Design review of the part built by this model. Coordinates are the model's own, in mm. Face numbers are marked on the shaded views. Round coordinates to 2 decimals unless told otherwise and drop trailing zeros. Write each loop counter-clockwise with the first axis right and the second up, starting at its lowest first coordinate (ties: lowest second). Pieces come first, ordered by that corner, then holes. Notation, with made-up numbers: (-10.75, -7) -> (33.25, -7) arc R18 ccw to (33.25, 18) -> close; hole circle Ø6 at (79.25, 74). An arc over 180 degrees is marked (long way). Write item = value, one per line. Start each with the question number.
Item 1: Add section C-C, the plane z = 124. State the section outline as (x, y) points.
Item 2: For pin 1 Ø1.5 at (x, z) = (16, 61.5) entering from +Y; pin 2 Ø3.5 at (x, z) = (-9.05, 111.48) entering from +Y; pin 3 Ø3 at (x, z) = (46.5, 136.5) entering from +Y; pin 4 Ø8 at (y, z) = (7.5, 117) entering from -X, all flat-tipped, find the tip position at first contact; note any pin that passes through.
Item 3: Add section B-B, the plane y = 19. State the section outline as (x, z) points (3 decimals).
Item 4: To check wall thickness, follow L1, parallel to Z at x = -45, y = 22 (3 decimals); L2, parallel to X at y = 1, z = 25 (3 decimals); L3, parallel to Y at x = 0, z = 69. State the ranges of each line that lie inside material, in increasing order.
Item 5: Add section A-A, the plane y = 7.5. State how many separate pieces and enclosed holes the cut face has, then the cut area to 3 significant figures.
Item 6: Mouldability with a two-part tool opening along Y and no side actions: class the marked faces 1 and 2 as released by +Y, released by -Y, zero draft, split by the parting line, or undercut.
Item 7: Add section D-D, the plane x = -27. State the section outline as (y, z) points.
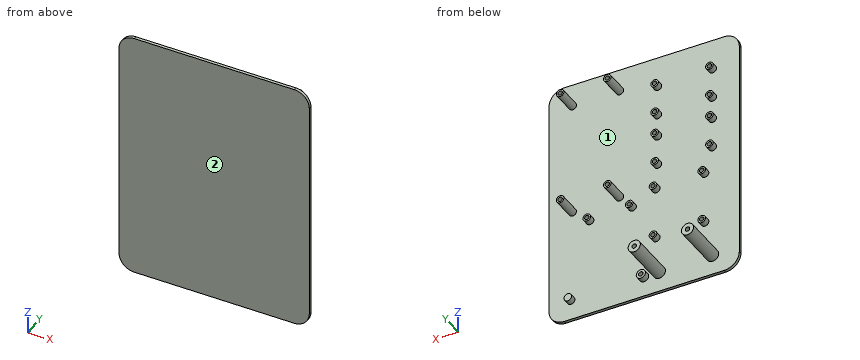
from build123d import *

# Parameters (mm, degrees)
SKETCH_1_R         = 2.5
EXTRUDE_1_DEPTH    = 4
SKETCH_1_R_2       = 3
EXTRUDE_1_2_DEPTH  = 4
EXTRUDE_1_3_DEPTH  = 4
EXTRUDE_1_4_DEPTH  = 4
EXTRUDE_1_5_DEPTH  = 4
EXTRUDE_1_6_DEPTH  = 4
EXTRUDE_1_7_DEPTH  = 4
EXTRUDE_1_8_DEPTH  = 4
EXTRUDE_1_9_DEPTH  = 4
EXTRUDE_1_10_DEPTH = 4
EXTRUDE_1_11_DEPTH = 4
EXTRUDE_1_12_DEPTH = 4
EXTRUDE_1_13_DEPTH = 4
EXTRUDE_1_14_DEPTH = 4
EXTRUDE_1_15_DEPTH = 4
EXTRUDE_1_16_DEPTH = 4
SKETCH_1_3_R       = 2.5
EXTRUDE_2_DEPTH    = 15
EXTRUDE_2_2_DEPTH  = 15
EXTRUDE_2_3_DEPTH  = 15
EXTRUDE_2_4_DEPTH  = 15
SKETCH_1_4_R       = 4
EXTRUDE_3_DEPTH    = 30
EXTRUDE_3_2_DEPTH  = 30
SKETCH_2_W         = 125
SKETCH_2_H         = 165
EXTRUDE_4_DEPTH    = 2
FILLET_1_R         = 10
SKETCH_9_W         = 1.475
SKETCH_9_H         = 30
MM_3_AT_2_COUNT    = 2
MM_3_AT_2_PITCH    = 56.007567425
MM_3_AT_3_COUNT    = 2
MM_3_AT_3_PITCH    = 72.159569674
MM_3_AT_4_COUNT    = 2
MM_3_AT_4_PITCH    = 52.22731905
MM_3_AT_5_COUNT    = 2
MM_3_AT_5_PITCH    = 37.325726715
MM_3_AT_6_COUNT    = 2
MM_3_AT_6_PITCH    = 17.717201651
MM_3_AT_7_COUNT    = 2
MM_3_AT_7_PITCH    = 34.5
MM_3_AT_8_COUNT    = 2
MM_3_AT_8_PITCH    = 59.709714453
MM_3_AT_9_COUNT    = 2
MM_3_AT_9_PITCH    = 66.635200908
MM_3_AT_10_COUNT   = 2
MM_3_AT_10_PITCH   = 71.695536821
MM_3_AT_11_COUNT   = 2
MM_3_AT_11_PITCH   = 75.871602066
MM_3_AT_12_COUNT   = 2
MM_3_AT_12_PITCH   = 86.987675624
MM_3_AT_13_COUNT   = 2
MM_3_AT_13_PITCH   = 116.476846242
MM_3_AT_14_COUNT   = 2
MM_3_AT_14_PITCH   = 95.586858976
MM_3_AT_15_COUNT   = 2
MM_3_AT_15_PITCH   = 78.355146818
MM_3_AT_16_COUNT   = 2
MM_3_AT_16_PITCH   = 60.49973878
MM_3_AT_17_COUNT   = 2
MM_3_AT_17_PITCH   = 48.22587907
MM_3_AT_18_COUNT   = 2
MM_3_AT_18_PITCH   = 35.304741489
MM_3_AT_19_COUNT   = 2
MM_3_AT_19_PITCH   = 32
MM_3_AT_20_COUNT   = 2
MM_3_AT_20_PITCH   = 48.187238975


with BuildPart() as part:
    # Sketch 1 → Extrude 1 (new body)
    with BuildSketch(Plane(origin=(0, 0, 0), x_dir=(1, 0, 0), z_dir=(0, 1, 0))):
        with Locations((-8, -25)):
            Circle(SKETCH_1_R)
    extrude(amount=EXTRUDE_1_DEPTH)



with BuildPart() as body_2:
    # Sketch 1 → Extrude 1 2 (new body)
    with BuildSketch(Plane(origin=(0, 0, 0), x_dir=(1, 0, 0), z_dir=(0, 1, 0))):
        Circle(SKETCH_1_R_2)
    extrude(amount=EXTRUDE_1_2_DEPTH)


with BuildPart() as body_3:
    # Sketch 1 → Extrude 1 3 (new body)
    with BuildSketch(Plane(origin=(0, 0, 0), x_dir=(1, 0, 0), z_dir=(0, 1, 0))):
        with Locations((-9.048256427, -96.482766011)):
            Circle(SKETCH_1_R)
    extrude(amount=EXTRUDE_1_3_DEPTH)


with BuildPart() as body_4:
    # Sketch 1 → Extrude 1 4 (new body)
    with BuildSketch(Plane(origin=(0, 0, 0), x_dir=(1, 0, 0), z_dir=(0, 1, 0))):
        with Locations((-45.048256427, -96.482766011)):
            Circle(SKETCH_1_R)
    extrude(amount=EXTRUDE_1_4_DEPTH)


with BuildPart() as body_5:
    # Sketch 1 → Extrude 1 5 (new body)
    with BuildSketch(Plane(origin=(0, 0, 0), x_dir=(1, 0, 0), z_dir=(0, 1, 0))):
        with Locations((-45.048256427, -76.482766011)):
            Circle(SKETCH_1_R)
    extrude(amount=EXTRUDE_1_5_DEPTH)


with BuildPart() as body_6:
    # Sketch 1 → Extrude 1 6 (new body)
    with BuildSketch(Plane(origin=(0, 0, 0), x_dir=(1, 0, 0), z_dir=(0, 1, 0))):
        with Locations((-9.048256427, -76.482766011)):
            Circle(SKETCH_1_R)
    extrude(amount=EXTRUDE_1_6_DEPTH)


with BuildPart() as body_7:
    # Sketch 1 → Extrude 1 7 (new body)
    with BuildSketch(Plane(origin=(0, 0, 0), x_dir=(1, 0, 0), z_dir=(0, 1, 0))):
        with Locations((-45.048256427, -131.482766011)):
            Circle(SKETCH_1_R)
    extrude(amount=EXTRUDE_1_7_DEPTH)


with BuildPart() as body_8:
    # Sketch 1 → Extrude 1 8 (new body)
    with BuildSketch(Plane(origin=(0, 0, 0), x_dir=(1, 0, 0), z_dir=(0, 1, 0))):
        with Locations((-45.048256427, -111.482766011)):
            Circle(SKETCH_1_R)
    extrude(amount=EXTRUDE_1_8_DEPTH)


with BuildPart() as body_9:
    # Sketch 1 → Extrude 1 9 (new body)
    with BuildSketch(Plane(origin=(0, 0, 0), x_dir=(1, 0, 0), z_dir=(0, 1, 0))):
        with Locations((-9.048256427, -111.482766011)):
            Circle(SKETCH_1_R)
    extrude(amount=EXTRUDE_1_9_DEPTH)


with BuildPart() as body_10:
    # Sketch 1 → Extrude 1 10 (new body)
    with BuildSketch(Plane(origin=(0, 0, 0), x_dir=(1, 0, 0), z_dir=(0, 1, 0))):
        with Locations((-40, -59.5)):
            Circle(SKETCH_1_R)
    extrude(amount=EXTRUDE_1_10_DEPTH)


with BuildPart() as body_11:
    # Sketch 1 → Extrude 1 11 (new body)
    with BuildSketch(Plane(origin=(0, 0, 0), x_dir=(1, 0, 0), z_dir=(0, 1, 0))):
        with Locations((-8, -59.5)):
            Circle(SKETCH_1_R)
    extrude(amount=EXTRUDE_1_11_DEPTH)


with BuildPart() as body_12:
    # Sketch 1 → Extrude 1 12 (new body)
    with BuildSketch(Plane(origin=(0, 0, 0), x_dir=(1, 0, 0), z_dir=(0, 1, 0))):
        with Locations((48, 0)):
            Circle(SKETCH_1_R)
    extrude(amount=EXTRUDE_1_12_DEPTH)


with BuildPart() as body_13:
    # Sketch 1 → Extrude 1 13 (new body)
    with BuildSketch(Plane(origin=(0, 0, 0), x_dir=(1, 0, 0), z_dir=(0, 1, 0))):
        with Locations((-9.048256427, -131.482766011)):
            Circle(SKETCH_1_R)
    extrude(amount=EXTRUDE_1_13_DEPTH)


with BuildPart() as body_14:
    # Sketch 1 → Extrude 1 14 (new body)
    with BuildSketch(Plane(origin=(0, 0, 0), x_dir=(1, 0, 0), z_dir=(0, 1, 0))):
        with Locations((7.6, -52)):
            Circle(SKETCH_1_R)
    extrude(amount=EXTRUDE_1_14_DEPTH)


with BuildPart() as body_15:
    # Sketch 1 → Extrude 1 15 (new body)
    with BuildSketch(Plane(origin=(0, 0, 0), x_dir=(1, 0, 0), z_dir=(0, 1, 0))):
        with Locations((35.5, -52)):
            Circle(SKETCH_1_R)
    extrude(amount=EXTRUDE_1_15_DEPTH)


with BuildPart() as body_16:
    # Sketch 1 → Extrude 1 16 (new body)
    with BuildSketch(Plane(origin=(0, 0, 0), x_dir=(1, 0, 0), z_dir=(0, 1, 0))):
        with Locations((-40, -25)):
            Circle(SKETCH_1_R)
    extrude(amount=EXTRUDE_1_16_DEPTH)


with BuildPart() as body_17:
    # Sketch 1_3 → Extrude 2 (new body)
    with BuildSketch(Plane(origin=(0, 0, 0), x_dir=(1, 0, 0), z_dir=(0, 1, 0))):
        with Locations((15.951743573, -137)):
            Circle(SKETCH_1_3_R)
    extrude(amount=EXTRUDE_2_DEPTH)


with BuildPart() as body_18:
    # Sketch 1_3 → Extrude 2 2 (new body)
    with BuildSketch(Plane(origin=(0, 0, 0), x_dir=(1, 0, 0), z_dir=(0, 1, 0))):
        with Locations((46.951743573, -137)):
            Circle(SKETCH_1_3_R)
    extrude(amount=EXTRUDE_2_2_DEPTH)


with BuildPart() as body_19:
    # Sketch 1_3 → Extrude 2 3 (new body)
    with BuildSketch(Plane(origin=(0, 0, 0), x_dir=(1, 0, 0), z_dir=(0, 1, 0))):
        with Locations((46.951743573, -62)):
            Circle(SKETCH_1_3_R)
    extrude(amount=EXTRUDE_2_3_DEPTH)


with BuildPart() as body_20:
    # Sketch 1_3 → Extrude 2 4 (new body)
    with BuildSketch(Plane(origin=(0, 0, 0), x_dir=(1, 0, 0), z_dir=(0, 1, 0))):
        with Locations((15.951743573, -62)):
            Circle(SKETCH_1_3_R)
    extrude(amount=EXTRUDE_2_4_DEPTH)


with BuildPart() as body_21:
    # Sketch 1_4 → Extrude 3 (new body)
    with BuildSketch(Plane(origin=(0, 0, 0), x_dir=(1, 0, 0), z_dir=(0, 1, 0))):
        with Locations((-45, 0)):
            Circle(SKETCH_1_4_R)
    extrude(amount=EXTRUDE_3_DEPTH)


with BuildPart() as body_22:
    # Sketch 1_4 → Extrude 3 2 (new body)
    with BuildSketch(Plane(origin=(0, 0, 0), x_dir=(1, 0, 0), z_dir=(0, 1, 0))):
        with Locations((-10, 0)):
            Circle(SKETCH_1_4_R)
    extrude(amount=EXTRUDE_3_2_DEPTH)


with BuildPart() as part_1:
    add(part.part)

    add(body_2.part)  # Extrude 4 merges body 2

    add(body_3.part)  # Extrude 4 merges body 3

    add(body_4.part)  # Extrude 4 merges body 4

    add(body_5.part)  # Extrude 4 merges body 5

    add(body_6.part)  # Extrude 4 merges body 6

    add(body_7.part)  # Extrude 4 merges body 7

    add(body_8.part)  # Extrude 4 merges body 8

    add(body_9.part)  # Extrude 4 merges body 9

    add(body_10.part)  # Extrude 4 merges body 10

    add(body_11.part)  # Extrude 4 merges body 11

    add(body_12.part)  # Extrude 4 merges body 12

    add(body_13.part)  # Extrude 4 merges body 13

    add(body_14.part)  # Extrude 4 merges body 14

    add(body_15.part)  # Extrude 4 merges body 15

    add(body_16.part)  # Extrude 4 merges body 16

    add(body_17.part)  # Extrude 4 merges body 17

    add(body_18.part)  # Extrude 4 merges body 18

    add(body_19.part)  # Extrude 4 merges body 19

    add(body_20.part)  # Extrude 4 merges body 20

    add(body_21.part)  # Extrude 4 merges body 21

    add(body_22.part)  # Extrude 4 merges body 22
    # Sketch 2 → Extrude 4 (add)
    with BuildSketch(Plane(origin=(0, 0, 0), x_dir=(1, 0, 0), z_dir=(0, 1, 0))):
        with Locations((0, -69.425835086)):
            Rectangle(SKETCH_2_W, SKETCH_2_H)
    extrude(amount=-EXTRUDE_4_DEPTH)

    # Fillet 1
    fillet_1_edges = [part_1.edges().sort_by_distance(p)[0] for p in [
        (62.5, -1, -13.074164914),
        (62.5, -1, 151.925835086),
        (-62.5, -1, 151.925835086),
        (-62.5, -1, -13.074164914),
    ]]
    fillet(fillet_1_edges, radius=FILLET_1_R)

    # Sketch 9 → mm _3 (revolve, cut)
    with BuildSketch(Plane(origin=(-40, 0, 59.5), x_dir=(0, 0, -1), z_dir=(1, 0, 0))):
        with Locations((0.7375, 15)):
            Rectangle(SKETCH_9_W, SKETCH_9_H)
    mm_3 = revolve(axis=Axis((-40, -6.35, 59.5), (0, 1, 0)), mode=Mode.SUBTRACT)

    # mm _3 at 2: mm _3 ×2
    with Locations(*[Vector(0.99900328, 0, 0.044636825) * (i * MM_3_AT_2_PITCH) for i in range(1, MM_3_AT_2_COUNT)]):
        add(mm_3, mode=Mode.SUBTRACT)

    # mm _3 at 3: mm _3 ×2
    with Locations(*[Vector(-0.069959625, 0, 0.997549824) * (i * MM_3_AT_3_PITCH) for i in range(1, MM_3_AT_3_COUNT)]):
        add(mm_3, mode=Mode.SUBTRACT)

    # mm _3 at 4: mm _3 ×2
    with Locations(*[Vector(-0.096659306, 0, 0.995317526) * (i * MM_3_AT_4_PITCH) for i in range(1, MM_3_AT_4_COUNT)]):
        add(mm_3, mode=Mode.SUBTRACT)

    # mm _3 at 5: mm _3 ×2
    with Locations(*[Vector(-0.135248711, 0, 0.99081168) * (i * MM_3_AT_5_PITCH) for i in range(1, MM_3_AT_5_COUNT)]):
        add(mm_3, mode=Mode.SUBTRACT)

    # mm _3 at 6: mm _3 ×2
    with Locations(*[Vector(-0.284935315, 0, 0.958546747) * (i * MM_3_AT_6_PITCH) for i in range(1, MM_3_AT_6_COUNT)]):
        add(mm_3, mode=Mode.SUBTRACT)

    # mm _3 at 7: mm _3 ×2
    with Locations(*[(0, 0, -i * MM_3_AT_7_PITCH) for i in range(1, MM_3_AT_7_COUNT)]):
        add(mm_3, mode=Mode.SUBTRACT)

    # mm _3 at 8: mm _3 ×2
    with Locations(*[Vector(-0.083738468, 0, -0.996487767) * (i * MM_3_AT_8_PITCH) for i in range(1, MM_3_AT_8_COUNT)]):
        add(mm_3, mode=Mode.SUBTRACT)

    # mm _3 at 9: mm _3 ×2
    with Locations(*[Vector(0.450212494, 0, -0.892921447) * (i * MM_3_AT_9_PITCH) for i in range(1, MM_3_AT_9_COUNT)]):
        add(mm_3, mode=Mode.SUBTRACT)

    # mm _3 at 10: mm _3 ×2
    with Locations(*[Vector(0.557914785, 0, -0.829898242) * (i * MM_3_AT_10_PITCH) for i in range(1, MM_3_AT_10_COUNT)]):
        add(mm_3, mode=Mode.SUBTRACT)

    # mm _3 at 11: mm _3 ×2
    with Locations(*[Vector(0.995102225, 0, -0.098851214) * (i * MM_3_AT_11_PITCH) for i in range(1, MM_3_AT_11_COUNT)]):
        add(mm_3, mode=Mode.SUBTRACT)

    # mm _3 at 12: mm _3 ×2
    with Locations(*[Vector(0.999586929, 0, 0.028739703) * (i * MM_3_AT_12_PITCH) for i in range(1, MM_3_AT_12_COUNT)]):
        add(mm_3, mode=Mode.SUBTRACT)

    # mm _3 at 13: mm _3 ×2
    with Locations(*[Vector(0.746515264, 0, 0.66536829) * (i * MM_3_AT_13_PITCH) for i in range(1, MM_3_AT_13_COUNT)]):
        add(mm_3, mode=Mode.SUBTRACT)

    # mm _3 at 14: mm _3 ×2
    with Locations(*[Vector(0.585349745, 0, 0.810780905) * (i * MM_3_AT_14_PITCH) for i in range(1, MM_3_AT_14_COUNT)]):
        add(mm_3, mode=Mode.SUBTRACT)

    # mm _3 at 15: mm _3 ×2
    with Locations(*[Vector(0.395018641, 0, 0.918673105) * (i * MM_3_AT_15_PITCH) for i in range(1, MM_3_AT_15_COUNT)]):
        add(mm_3, mode=Mode.SUBTRACT)

    # mm _3 at 16: mm _3 ×2
    with Locations(*[Vector(0.511601276, 0, 0.859222983) * (i * MM_3_AT_16_PITCH) for i in range(1, MM_3_AT_16_COUNT)]):
        add(mm_3, mode=Mode.SUBTRACT)

    # mm _3 at 17: mm _3 ×2
    with Locations(*[Vector(0.641807763, 0, 0.766865565) * (i * MM_3_AT_17_PITCH) for i in range(1, MM_3_AT_17_COUNT)]):
        add(mm_3, mode=Mode.SUBTRACT)

    # mm _3 at 18: mm _3 ×2
    with Locations(*[Vector(0.876702173, 0, 0.481033575) * (i * MM_3_AT_18_PITCH) for i in range(1, MM_3_AT_18_COUNT)]):
        add(mm_3, mode=Mode.SUBTRACT)

    # mm _3 at 19: mm _3 ×2
    with Locations(*[(i * MM_3_AT_19_PITCH, 0, 0) for i in range(1, MM_3_AT_19_COUNT)]):
        add(mm_3, mode=Mode.SUBTRACT)

    # mm _3 at 20: mm _3 ×2
    with Locations(*[Vector(0.987813392, 0, -0.155642866) * (i * MM_3_AT_20_PITCH) for i in range(1, MM_3_AT_20_COUNT)]):
        add(mm_3, mode=Mode.SUBTRACT)

    # Sketch 10 → mm _3 2 (revolve, cut)
    with BuildSketch(Plane(origin=(-8, 0, 25), x_dir=(0, 0, -1), z_dir=(1, 0, 0))):
        Polygon((0, 0), (0, 30), (1.475, 30), (1.475, 0.05), (1.525, 0), align=None)
    revolve(axis=Axis((-8, -6.35, 25), (0, 1, 0)), mode=Mode.SUBTRACT)


solid = part_1.part
Result set:
q1.outline = (-62.5, -2) -> (62.5, -2) -> (62.5, 0) -> (-62.5, 0) -> close
q2.pin_1 = 0
q2.pin_2 = 4
q2.pin_3 = 15
q2.pin_4 = through
q3.outline = circle Ø8 at (-45, 0); circle Ø8 at (-10, 0); hole circle Ø2.95 at (-45, 0); hole circle Ø2.95 at (-10, 0)
q4.L1 = -4 to -1.475, 1.475 to 4
q4.L2 = -42.5 to -41.475, -38.525 to -37.5, -10.5 to -9.475, -6.525 to -5.5
q4.L3 = -2 to 0
q5.separate_pieces = 6
q5.enclosed_holes = 6
q5.area = 138 mm²
q6.face_1 = released by +Y
q6.face_2 = released by -Y
q7.outline = (-2, -13.07) -> (0, -13.07) -> (0, 151.93) -> (-2, 151.93) -> close
